Autodesk Inventor part; units mm, degrees
ref_plane "YZ Plane" through (0, 0, 0) normal (1, 0, 0) x (0, 1, 0)
ref_plane "XZ Plane" through (0, 0, 0) normal (0, 1, 0) x (-1, 0, 0)
ref_plane "XY Plane" through (0, 0, 0) normal (0, 0, 1) x (1, 0, 0)
sketch "Sketch4" plane through (0, 0, 0) normal (0, 0, 1) x (1, 0, 0)
  line L0 (0, 0) -> (7.3, 0)
  line L1 (7.3, 0) -> (7.3, 22.5)
  line L2 (7.3, 22.5) -> (0.3, 22.5)
  line L3 (0.3, 22.5) -> (0.3, 14)
  line L4 (0.3, 14) -> (1.5, 14)
  line L5 (1.5, 14) -> (1.5, 12.5)
  line L6 (1.5, 12.5) -> (0, 12.5)
  line L7 (0, 12.5) -> (0, 7.5)
  line L8 (0, 7.5) -> (0, 7.5)
  line L9 (0, 7.5) -> (0, 0)
  dimension "d44" = 25
  dimension "d45" = 1.5
  dimension "d46" = 1.2
  dimension "d47" = 1.5
  dimension "d53" = 45
  dimension "d58" = 7
  dimension "d59" = 15
  dimension "d60" = 0
revolve "Revolution2" add sketch "Sketch4" angle 360 about axis through (0, 0, 0) along (1, 0, 0)
sketch "Sketch7" plane through (7.3, 0, 0) normal (1, 0, 0) x (0, 0, -1)
  line L0 (-20, 26) -> (20, 26)
  line L1 (20, 26) -> (20, 16)
  line L2 (20, 16) -> (-20, 16)
  line L3 (-20, 16) -> (-20, 26)
  line L4 (20, -16) -> (-20, -16)
  line L5 (-20, -16) -> (-20, -26)
  line L6 (-20, -26) -> (20, -26)
  line L7 (20, -26) -> (20, -16)
  point P0 (0, 0)
  point P1 (0, 16)
  point P2 (0, -16)
  dimension "d61" = 16
  dimension "d62" = 16
  dimension "d63" = 10
  dimension "d64" = 10
  dimension "d65" = 20
extrude "Extrusion2" cut sketch "Sketch7" against normal blind 20
sketch "Sketch10" plane through (0, 0, 0) normal (-1, 0, 0) x (0, 0, 1)
  circle A0 centre (0, 0) radius 12.5
  circle A1 centre (0, 0) radius 12.5
  line L0 (-12.5, 0) -> (12.5, 0) construction
  line L1 (-12.4984, 0.2) -> (12.4984, 0.2)
  line L2 (-12.0835, 3.2) -> (12.0835, 3.2)
  point P0 (-12.4984, 0.2)
  point P1 (12.4984, 0.2)
  dimension "d72" = 0.2
  dimension "d73" = 3
extrude "Extrusion4" add sketch "Sketch10" along normal blind 26 contours L1 A0 L2
sketch "Sketch11" plane through (0, 3.2, 12.0835) normal (0, 1, 0) x (1, 0, 0)
  circle A0 centre (-8, 12.0835) radius 5 construction
  circle A1 centre (-8, 12.0835) radius 7
  point P0 (0, 12.0835)
  dimension "d76" = 14
extrude "Extrusion5" cut sketch "Sketch11" against normal through all
sketch "Sketch12" plane through (0, 0, 0) normal (-1, 0, 0) x (0, 0, 1)
  line L0 (12.4984, 0.2) -> (-12.4984, 0.2)
  arc A0 (-12.4984, 0.2) -> (12.4984, 0.2) centre (0, 0) ccw
  line L1 (-6, 0.2) -> (-6, -10.9659)
  circle A1 centre (0, 0) radius 12.5
  line L2 (12.4984, 0.2) -> (-12.4984, 0.2)
  line L3 (6, 0.2) -> (6, -10.9659)
  line L4 (-12.4984, 0.2) -> (12.4984, 0.2)
  dimension "d79" = 6
  dimension "d80" = 6
extrude "Extrusion6" add sketch "Sketch12" along normal blind 26 contours A0 L3 L0 | L0 L1 A0
sketch "Sketch13" plane through (7.3, 0, 0) normal (1, 0, 0) x (0, 0, -1)
  circle A0 centre (0, 0) radius 12.5
  circle A1 centre (0, 0) radius 10
  dimension "d83" = 20
extrude "Extrusion7" cut sketch "Sketch13" against normal blind 15 contours A1
sketch "Sketch14" plane through (7.3, 0, 0) normal (1, 0, 0) x (0, 0, -1)
  circle A0 centre (0, 0) radius 12.5
  circle A1 centre (0, 0) radius 14.5
  dimension "d86" = 2
extrude "Extrusion8" cut sketch "Sketch14" against normal blind 1.2
sketch "Sketch15" plane through (7.3, 0, 0) normal (1, 0, 0) x (0, 0, -1)
  line L0 (0, 0) -> (12.7279, -12.7279)
  line L1 (0, 0) -> (18, 0) construction
  dimension "d89" = 18
  dimension "d90" = 45
hole "Hole3" at (7.3, -12.7279, -12.7279) direction (-1, 0, 0) diameter 3.4 end through all
pattern_circular "Circular Pattern2" count 4 over 360 about axis through (0.75, 0, 0) along (1, 0, 0) of "Hole3"
equation "\"d64\" = d63"
properties part number "022" material "Aluminum 6061"
Here's how the part is built. I have some questions about the finished solid (model axes, mm). A direction names the side the tool comes from. Round coordinates to 2 decimals unless told otherwise and drop trailing zeros. Write each loop counter-clockwise with the first axis right and the second up, starting at its lowest first coordinate (ties: lowest second). Pieces come first, ordered by that corner, then holes.
1. Suppose I cut it at A-A (z = -1). List the corners of the cut face in (x, y) for me, and give its area (3 significant figures).
2. I need wall thicknesses on L1, parallel to Z at x = 1, y = 0; L2, parallel to Z at x = 0, y = 0; L3, parallel to Y at x = -17, z = 3. Which ranges of each line are inside material? Lowest first, please.
3. If we mould it in two halves opening along Z, with no side actions, what happens to faces 1 (the flat face through (-16, 3.2, 0)), 2 (the cylindrical face through (6.708, -12.864, -6.691)), 3 (the flat face through (-9.2, 0.2, -6.4)), 4 (the cylindrical face through (3.8, -0.2, 22.5))? For each: released by +Z, released by -Z, zero draft, split by the parting line, or undercut.
4. Suppose I cut it at B-B (x = -5). List the corners of the cut face in (y, z) for me.
5. Suppose I cut it at D-D (x = 4.5). List the corners of the cut face in (y, z) for me, and give its area (3 significant figures).
6. Will these pins go through, and if not, where does the flat tip stop? pin 1 Ø3.5 at (x, y) = (-17.5, -7.5) entering from +Z; pin 2 Ø3 at (x, y) = (-3, -12) entering from -Z; pin 3 Ø0.5 at (x, z) = (-10.5, 6.5) entering from +Y.
7. Suppose I cut it at C-C (y = -3). List the corners of the cut face in (x, z) for me, and give its area (3 significant figures).
8. For faces 5 (the flat face through (-16, -5, -6)), 6 (the flat face through (-9.2, 0.2, 6.4)), 7 (the flat face through (0, -11, 0)), which set-ups out of +Z, -Z, +X, -X, +Y, -Y let a thin tool reach every point of the face, with its end or its side?
Answer sheet:
1. outline: (-26, 0.2) - (-14.93, 0.2) - (-14.93, 3.2) - (-26, 3.2) - close; (0, -12.46) - (1.5, -12.46) - (1.5, -13.96) - (0.3, -13.96) - (0.3, -16) - (7.3, -16) - (7.3, -14.47) - (6.1, -14.47) - (6.1, -12.46) - (7.3, -12.46) - (7.3, -9.95) - (0, -9.95) - close; (0, 9.95) - (7.3, 9.95) - (7.3, 12.46) - (6.1, 12.46) - (6.1, 14.47) - (7.3, 14.47) - (7.3, 16) - (0.3, 16) - (0.3, 13.96) - (1.5, 13.96) - (1.5, 12.46) - (0, 12.46) - close
1. area: 111 mm2
2. L1: z = -22.5 to -14, -12.5 to -10, 10 to 12.5, 14 to 22.5
2. L2: z = -12.5 to -10, 10 to 12.5
2. L3: y = 0.2 to 3.2
3. face 1: zero draft
3. face 2: undercut
3. face 3: undercut
3. face 4: released by +Z
4. outline: (-10.97, -6) arc R12.5 ccw to (3.2, -12.08) - (3.2, -9.47) arc R10 cw to (-8, -6) - close; (-10.97, 6) - (-8, 6) arc R10 cw to (3.2, 9.47) - (3.2, 12.08) arc R12.5 ccw to start
5. outline: (-16, -15.82) arc R22.5 ccw to (16, -15.82) - (16, 15.82) arc R22.5 ccw to (-16, 15.82) - close; hole circle Ø3.4 at (-12.73, -12.73); hole circle Ø3.4 at (-12.73, 12.73); hole circle Ø20 at (0, 0); hole circle Ø3.4 at (12.73, -12.73); hole circle Ø3.4 at (12.73, 12.73)
5. area: 957 mm2
6. pin 1: stops at z = 11.1
6. pin 2: stops at z = -6.78
6. pin 3: stops at y = 3.2
7. outline: (-26, -12.13) - (1.5, -12.13) - (1.5, -13.67) - (0.3, -13.67) - (0.3, -22.3) - (7.3, -22.3) - (7.3, -14.19) - (6.1, -14.19) - (6.1, -12.13) - (7.3, -12.13) - (7.3, -9.54) - (-7.7, -9.54) - (-7.7, -6) - (-26, -6) - close; (-26, 6) - (-7.7, 6) - (-7.7, 9.54) - (7.3, 9.54) - (7.3, 12.13) - (6.1, 12.13) - (6.1, 14.19) - (7.3, 14.19) - (7.3, 22.3) - (0.3, 22.3) - (0.3, 13.67) - (1.5, 13.67) - (1.5, 12.13) - (-26, 12.13) - close
7. area: 436 mm2
8. face 5: -X, -Y
8. face 6: +X, +Y
8. face 7: -X, +Y, -Y
